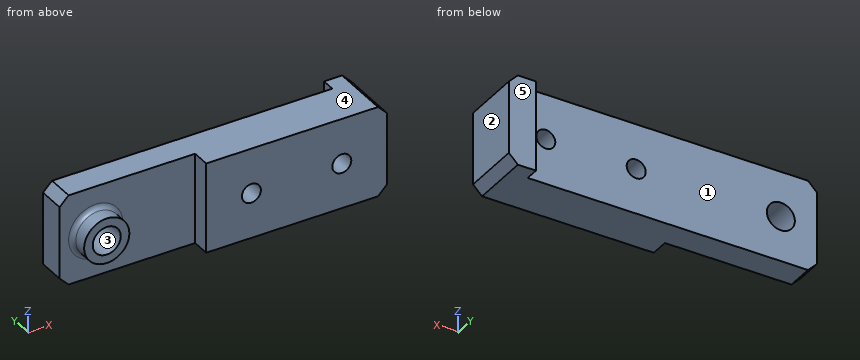
from build123d import *

# Parameters (mm, degrees)
EXTRUDE_1_DEPTH     = 10
SKETCH_3_R          = 5
EXTRUDE_2_DEPTH     = 4
CHAMFER_1_SIZE      = 2
CHAMFER_2_SIZE      = 2
SKETCH_4_R          = 2.1
SKETCH_4_R_2        = 3.1
CUT_EXTRUDE_1_DEPTH = 72.895757872
FILLET_1_R          = 1


with BuildPart() as part:
    # 草图1 → 凸台-拉伸1 (new, symmetric)
    with BuildSketch(Plane.XY):
        Polygon((0, 6), (0, 12), (64, 12), (64, 15), (70, 15), (70, 12), (70, 2), (30, 2), (30, 6), align=None)
    extrude(amount=EXTRUDE_1_DEPTH, both=True)

    # 草图3 → 凸台-拉伸2 (add)
    with BuildSketch(Plane.XZ.offset(-6)):
        with Locations(Location((8, 0, 0), (0, 0, 90))):
            Circle(SKETCH_3_R)
    extrude(amount=EXTRUDE_2_DEPTH)

    # 倒角1
    chamfer_1_edges = [part.edges().sort_by_distance(p)[0] for p in [
        (0, 9, -10),
        (0, 9, 10),
    ]]
    chamfer(chamfer_1_edges, length=CHAMFER_1_SIZE)

    # 倒角2
    chamfer_2_edges = [part.edges().sort_by_distance(p)[0] for p in [
        (70, 8.5, 10),
        (70, 8.5, -10),
    ]]
    chamfer(chamfer_2_edges, length=CHAMFER_2_SIZE)

    # 草图4 → 切除-拉伸1 (cut, through all)
    with BuildSketch(Plane.XZ.offset(-2)):
        with Locations((40, 0)):
            Circle(SKETCH_4_R)
        with Locations((60, 0)):
            Circle(SKETCH_4_R)
        with Locations((8, 0)):
            Circle(SKETCH_4_R_2)
    extrude(amount=-CUT_EXTRUDE_1_DEPTH, mode=Mode.SUBTRACT)

    # 圆角1
    fillet_1_edges = [part.edges().sort_by_distance(p)[0] for p in [
        (8, 6, -5),
    ]]
    fillet(fillet_1_edges, radius=FILLET_1_R)


solid = part.part
Source: CAD feature listing. Evaluate the final solid. Frame: model axes, mm. Face numbers are marked on the shaded views. A direction names the side the tool comes from. Coordinates: 2 decimals unless noted, no trailing zeros. Loops run counter-clockwise (first coordinate to the right, second up) from the corner with the lowest first, then second, coordinate; pieces in that order, holes last. Notation, with made-up numbers: (47, 48) - (101, 48) arc R24 ccw to (101, 86) - close; hole circle Ø3 at (-6.75, -20.5). An arc over 180 degrees is marked (long way). One line per item, written item: value. Start each with the question number.
1. Set-up query: the marked faces 1 and 2. Return all of +Z, -Z, +X, -X, +Y, -Y with unobstructed straight access to the full face (end or side cutting, diameter ignored); none if empty.
2. Mould query, pull axis Z, two halves, no side actions, for the marked faces 3, 4 and 5. Classes: pulls with the +Z half, pulls with the -Z half, needs draft (parallel to the pull), parting line crosses it, or undercut.
3. Section B-B (z = 0). Return the cut outline in (x, y), and give its area (3 significant figures).
4. Section C-C (y = 6.75). Return the cut outline in (x, z).
5. Ray query, L1, parallel to X at y = 3.25, z = -0.25; L2, parallel to X at y = 7.75, z = -0.25; L3, parallel to Z at x = 8, y = 6.25. Return the intervals inside material, ascending.
6. Contact query for flat-ended pins moving along their axis: P1, Ø2.5, axis at y = 14, z = 0, coming from the -X side; P2, Ø5, axis at x = 15, z = 3, coming from the +Y side; P3, Ø10, axis at x = 21.5, z = 2, coming from the -Y side. Output: stop coordinate, or through.
7. Section A-A (x = 8). Return the cut outline in (y, z), and give its area (3 significant figures).
8. Section D-D (z = 8.75). Return the cut outline in (x, y), and give its area (3 significant figures).
Verdict:
1. face 1: +Z, -Z, -X, +Y
1. face 2: +Z, -Z, +X, +Y, -Y
2. face 3: undercut
2. face 4: pulls with the +Z half
2. face 5: needs draft
3. outline: (0, 6) - (2, 6) arc R1 cw to (3, 5) - (3, 2) - (4.9, 2) - (4.9, 12) - (0, 12) - close; (11.1, 2) - (13, 2) - (13, 5) arc R1 cw to (14, 6) - (30, 6) - (30, 2) - (37.9, 2) - (37.9, 12) - (11.1, 12) - close; (42.1, 2) - (57.9, 2) - (57.9, 12) - (42.1, 12) - close; (62.1, 2) - (70, 2) - (70, 15) - (64, 15) - (64, 12) - (62.1, 12) - close
3. area: 492 mm2
4. outline: (0, -8) - (2, -10) - (68, -10) - (70, -8) - (70, 8) - (68, 10) - (2, 10) - (0, 8) - close; hole circle Ø6.2 at (8, 0); hole circle Ø4.2 at (40, 0); hole circle Ø4.2 at (60, 0)
5. L1: x = 3.01 to 4.91, 11.09 to 12.99, 30 to 37.91, 42.09 to 57.91, 62.09 to 70
5. L2: x = 0 to 4.91, 11.09 to 37.91, 42.09 to 57.91, 62.09 to 70
5. L3: z = -10 to -3.1, 3.1 to 10
6. P1: stops at x = 64
6. P2: stops at y = 12
6. P3: stops at y = 6
7. outline: (2, -5) - (5, -5) arc R1 cw to (6, -6) - (6, -10) - (12, -10) - (12, -3.1) - (2, -3.1) - close; (2, 3.1) - (12, 3.1) - (12, 10) - (6, 10) - (6, 6) arc R1 cw to (5, 5) - (2, 5) - close
7. area: 98.4 mm2
8. outline: (0.75, 6) - (30, 6) - (30, 2) - (69.25, 2) - (69.25, 15) - (64, 15) - (64, 12) - (0.75, 12) - close
8. area: 584 mm2
